from build123d import *

# Parameters (mm, degrees)
EXTRUDE_1_DEPTH     = 50
SKETCH_4_R          = 3
CUT_EXTRUDE_1_DEPTH = 50
CHAMFER_1_SIZE      = 5
CHAMFER_2_SIZE      = 5
CHAMFER_4_SIZE      = 1
CHAMFER_5_SIZE      = 1
CHAMFER_6_SIZE      = 1


with BuildPart() as part:
    # 草图2 → 凸台-拉伸1 (new body)
    with BuildSketch(Plane.XY):
        Polygon((0, 0), (15, 0), (15, -5), (20, -10), (-20, -10), (-15, -5), (-15, 0), align=None)
    extrude(amount=EXTRUDE_1_DEPTH)

    # 草图4 → 切除-拉伸1 (cut)
    with BuildSketch(Plane.XZ.offset(10)):
        with Locations((0, 40)):
            Circle(SKETCH_4_R)
        with Locations((0, 10)):
            Circle(SKETCH_4_R)
    extrude(amount=-CUT_EXTRUDE_1_DEPTH, mode=Mode.SUBTRACT)

    # 倒角1
    chamfer_1_edges = [part.edges().sort_by_distance(p)[0] for p in [
        (-3, -10, 10),
    ]]
    chamfer(chamfer_1_edges, length=CHAMFER_1_SIZE)

    # 倒角2
    chamfer_2_edges = [part.edges().sort_by_distance(p)[0] for p in [
        (-3, -10, 40),
    ]]
    chamfer(chamfer_2_edges, length=CHAMFER_2_SIZE)

    # 倒角4
    chamfer_4_edges = [part.edges().sort_by_distance(p)[0] for p in [
        (15, 0, 25),
        (-15, 0, 25),
        (-3, 0, 40),
        (-3, 0, 10),
        (0, 0, 50),
        (0, 0, 0),
    ]]
    chamfer(chamfer_4_edges, length=CHAMFER_4_SIZE)

    # 倒角5
    chamfer_5_edges = [part.edges().sort_by_distance(p)[0] for p in [
        (20, -10, 25),
        (-20, -10, 25),
    ]]
    chamfer(chamfer_5_edges, length=CHAMFER_5_SIZE)

    # 倒角6
    chamfer_6_edges = [part.edges().sort_by_distance(p)[0] for p in [
        (0, -10, 0),
        (0, -10, 50),
    ]]
    chamfer(chamfer_6_edges, length=CHAMFER_6_SIZE)


solid = part.part
Read the model definition and answer for the solid it produces. Units are mm, in the model's axes. A direction names the side the tool comes from. Give positions to 0.01 mm unless a question says otherwise; leave off trailing zeros. Write each loop counter-clockwise with the first axis right and the second up, starting at its lowest first coordinate (ties: lowest second). Pieces come first, ordered by that corner, then holes. Notation, with made-up numbers: (42, 78) - (64, 78) arc R23 ccw to (64, 90) - close; hole circle Ø4 at (-33.75, -17.75). An arc over 180 degrees is marked (long way). Use CSV: the item, a comma, the result in double quotes. Start each with the question number.
(1) For faces 4 (the flat face through (15, -3, 25)), 5 (the conical face through (-0.72, -5.31, 6.77)), determine the directions among +Z, -Z, +X, -X, +Y, -Y from which every point of the face is accessible in a straight line to the end or side of a thin tool.
(2) Find section B-B (y = -8). Give the vertices of the cut face in (x, z).
(3) Find section A-A (z = 10). Give the vertices of the cut face in (x, y), plus the area to 3 significant figures.
(4) Consider line 1 along Z through (x, y) = (0, -2.7); line 2 along X through (y, z) = (-4.5, 14); line 3 along X through (y, z) = (-8.75, 43). Determine where each line is inside the solid, lowest interval first.
(5) Determine the mould class of faces 1 (the flat face through (-15, -3, 25)), 2 (the conical face through (1.496, -5.243, 37.123)), 3 (the flat face through (0.2, -0.5, 0.5)) for opening direction Z: +Z half, -Z half, draft (parallel to the pull), parting line (faces both ways), or undercut.
(6) Given P1, Ø5, axis at x = 0, z = 40, coming from the -Y side (3 decimals); P2, Ø8, axis at x = 0, z = 10, coming from the -Y side; P3, Ø5, axis at y = -8, z = 26.5, coming from the -X side; P4, Ø1.2, axis at y = -2, z = 31.5, coming from the -X side, each flat-ended and moving along its own axis, determine where each tip first touches the part or whether it passes through.
(7) Find section C-C (x = -0.5). Count the separate pieces of the cut face and the enclosed holes in it, plus the area to 3 significant figures.
Findings below:
1,face 4,"+Z, -Z, +X, +Y"
1,face 5,"-Y"
2,outline,"(-18, 0) - (18, 0) - (18, 50) - (-18, 50) - close; hole circle Ø12 at (0, 10); hole circle Ø12 at (0, 40)"
3,outline,"(-19.29, -9.29) - (-19, -10) - (-8, -10) - (-3, -5) - (-3, -1) - (-4, 0) - (-14, 0) - (-15, -1) - (-15, -5) - close; (3, -5) - (8, -10) - (19, -10) - (19.29, -9.29) - (15, -5) - (15, -1) - (14, 0) - (4, 0) - (3, -1) - close"
3,area,"237 mm2"
4,line 1,"0 to 7, 13 to 37, 43 to 50"
4,line 2,"-15 to 15"
4,line 3,"-18.75 to -6.05, 6.05 to 18.75"
5,face 1,"draft"
5,face 2,"undercut"
5,face 3,"-Z half"
6,P1,"through"
6,P2,"y = -6"
6,P3,"x = -19.29"
6,P4,"x = -15"
7,separate pieces,"3"
7,enclosed holes,"0"
7,area,"327 mm2"
